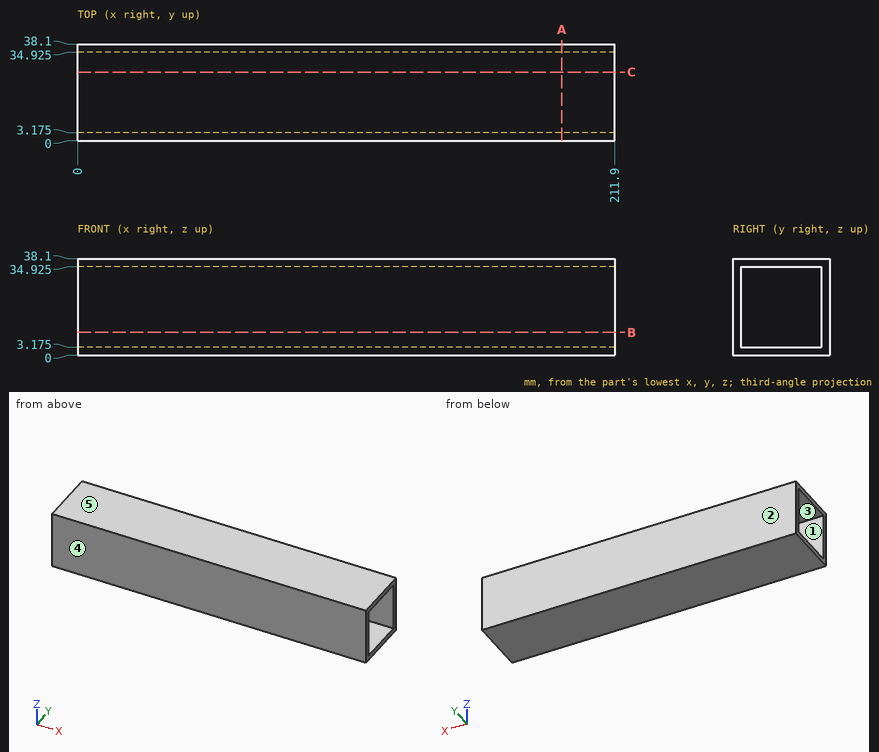
Study the drawing (mm; zero at the part's minimum x, y, z) and answer. A direction names the side the tool comes from. Give positions to 0.01 mm unless a question says otherwise; leave off trailing zeros. Order: outer loops, then holes, each group sorted by start corner. A loop starts at its lowest first (then second) coordinate and runs counter-clockwise, first axis right, second up. Notation, with made-up numbers: (73, 56) - (101, 56) arc R22 ccw to (101, 85) - close; hole circle Ø11 at (76.25, -15). An arc over 180 degrees is marked (long way). Answer as CSV lines item,"result". Start each with the question number.
Q1. Find the intervals of material crossed by L1, parallel to Z at x = 24, y = 6.5 (3 decimals), in increasing order. Write a range as [from, to].
Q2. For the marked faces 1 and 2, determine the directions among +Z, -Z, +X, -X, +Y, -Y from which every point of the face is accessible in a straight line to the end or side of a thin tool.
Q3. The part is cut by section B-B (z = 9). Write down the section's boundary in (x, y) (3 decimals), then the cut area to 3 significant figures.
Q4. The part is cut by section A-A (x = 191). Write down the section's boundary in (y, z) (3 decimals).
Q5. The mould has two halves that part along Y. Classify the marked faces 3, 4 and 5: +Y half, -Y half, draft (parallel to the pull), parting line (faces both ways), or undercut.
Check result:
1,L1,"z = [0, 3.175], [34.925, 38.1]"
2,face 1,"+X, -X"
2,face 2,"+Z, -Z, +X, -X, +Y"
3,outline,"(0, 0) - (211.9, 0) - (211.9, 3.175) - (0, 3.175) - close; (0, 34.925) - (211.9, 34.925) - (211.9, 38.1) - (0, 38.1) - close"
3,area,"1,350 mm²"
4,outline,"(0, 0) - (38.1, 0) - (38.1, 38.1) - (0, 38.1) - close; hole (3.175, 3.175) - (34.925, 3.175) - (34.925, 34.925) - (3.175, 34.925) - close"
5,face 3,"undercut"
5,face 4,"-Y half"
5,face 5,"draft"
